```python
from build123d import *

# Parameters (mm, degrees)
SKIZZE1_W                                           = 100
SKIZZE1_H                                           = 50
AUFSATZ_LINEAR_AUSTRAGEN1_DEPTH                     = 120
KERNLOCH_F_R_M8_HELICOIL1_D                         = 8.3
KERNLOCH_F_R_M8_HELICOIL1_DEPTH                     = 20
KERNLOCH_F_R_M8_HELICOIL1_TIP                       = 2.493571569
STIRNSENKUNG_F_R_M8_SENKSCHRAUBE_KOPF_B_D           = 9
STIRNSENKUNG_F_R_M8_SENKSCHRAUBE_KOPF_B_CBORE_D     = 15
STIRNSENKUNG_F_R_M8_SENKSCHRAUBE_KOPF_B_CBORE_DEPTH = 116


with BuildPart() as part:
    # Skizze1 → Aufsatz-Linear austragen1 (new body)
    with BuildSketch(Plane.XY):
        Rectangle(SKIZZE1_W, SKIZZE1_H)
    extrude(amount=AUFSATZ_LINEAR_AUSTRAGEN1_DEPTH)

    # Kernloch für M8 Helicoil1
    with Locations(Plane(origin=(0, 25, 0), x_dir=(1, 0, 0), z_dir=(0, 1, 0))):
        with Locations((35, -105), (-35, -15)):
            Hole(KERNLOCH_F_R_M8_HELICOIL1_D / 2, depth=KERNLOCH_F_R_M8_HELICOIL1_DEPTH)
            with Locations((0, 0, -(KERNLOCH_F_R_M8_HELICOIL1_DEPTH + KERNLOCH_F_R_M8_HELICOIL1_TIP / 2))):  # 118° drill point
                Cone(0, KERNLOCH_F_R_M8_HELICOIL1_D / 2, KERNLOCH_F_R_M8_HELICOIL1_TIP, mode=Mode.SUBTRACT)

    # Stirnsenkung für M8 Senkschraube (Kopf Button)1 (through all)
    with Locations(Plane.XY.offset(120)):
        with Locations((4.444e-06, 5)):
            CounterBoreHole(STIRNSENKUNG_F_R_M8_SENKSCHRAUBE_KOPF_B_D / 2, STIRNSENKUNG_F_R_M8_SENKSCHRAUBE_KOPF_B_CBORE_D / 2, STIRNSENKUNG_F_R_M8_SENKSCHRAUBE_KOPF_B_CBORE_DEPTH)


solid = part.part
```
Work out the finished part from the listing and answer in its coordinate system (mm). A direction names the side the tool comes from. Coordinates: 2 decimals unless noted, no trailing zeros. Order: outer loops, then holes, each group sorted by start corner. A loop starts at its lowest first (then second) coordinate and runs counter-clockwise, first axis right, second up. Notation, with made-up numbers: M 34.25,73 L 83.25,73 A23 ccw 83.25,104 Z; hole C -1.75,46 d6. An arc over 180 degrees is marked long. Use CSV: the item, a comma, the result in double quotes.
1) Consider line 1 (Z direction, x = 35, y = 20.5); line 2 (X direction, y = 19, z = 105); line 3 (Y direction, x = 5.5, z = 88). Determine where each line is inside the solid, lowest interval first. Write a range as [from, to].
Worked out:
line 1,"z = [0, 100.85], [109.15, 120]"
line 2,"x = [-50, 30.85], [39.15, 50]"
line 3,"y = [-25, -0.1], [10.1, 25]"
2) Section B-B on x = -6 is taken. Write down the section's boundary in (y, z), plus the area to 3 significant figures.
Worked out:
outline,"M -25,0 L 25,0 L 25,120 L 9.5,120 L 9.5,4 L 0.5,4 L 0.5,120 L -25,120 Z"
area,"4,960 mm^2"
3) For faces 1 (the face through (5, 5, 4)), 2 (the face through (-38.834, 14.86, 16.589)), 3 (the face through (0.98, 0.61, 1.97)), determine the directions among +Z, -Z, +X, -X, +Y, -Y from which every point of the face is accessible in a straight line to the end or side of a thin tool.
Worked out:
face 1,"+Z"
face 2,"+Y"
face 3,"+Z, -Z"
4) Determine the mould class of faces 4 (the face through (-1, 0, 0)), 5 (the face through (50, 0, 59)), 6 (the face through (-50, 0, 59)), 7 (the face through (-35.57, 2.94, 15.44)) for opening direction X: released by +X, released by -X, zero draft, split by the parting line, or undercut.
Worked out:
face 4,"zero draft"
face 5,"released by +X"
face 6,"released by -X"
face 7,"undercut"
5) Flat-ended cylindrical pins translate along their axes: pin 1 Ø7.5 at (x, z) = (-35, 15) entering from +Y; pin 2 Ø1.5 at (x, y) = (3.5, -3.5) entering from -Z; pin 3 Ø4.5 at (x, y) = (3, 2.5) entering from +Z; pin 4 Ø7 at (x, y) = (0, 5) entering from +Z. Find the tip coordinate at first contact, or state that the pin passes through.
Worked out:
pin 1,"stops at y = 4.76"
pin 2,"stops at z = 0"
pin 3,"stops at z = 4"
pin 4,"passes through"
6) Section A-A on z = 90.5 is taken. Write down the section's boundary in (x, y), plus the area to 3 significant figures.
Worked out:
outline,"M -50,-25 L 50,-25 L 50,25 L -50,25 Z; hole C 0,5 d15"
area,"4,820 mm^2"
